from build123d import *

# Parameters (mm, degrees)
F0_W     = 30
F0_H     = 22
F1_DEPTH = 1
F2_R     = 3
F3_R     = 4.5


with BuildPart() as f1:
    # F0 (on Top) → F1 (new body)
    with BuildSketch(Plane.XY):
        Rectangle(F0_W, F0_H)
        Polygon((7.75, 9.5), (13.5, 9.5), (13.5, 3.937851), (13.5, -9.5), (-13.5, -9.5), (-13.5, 3.937851), (-13.5, 9.5), (-7.75, 9.5), align=None, mode=Mode.SUBTRACT)
        Polygon((-13.5, 3.937851), (-7.75, 9.5), (-13.5, 9.5), align=None)
        Polygon((13.5, 3.937851), (13.5, 9.5), (7.75, 9.5), align=None)
    extrude(amount=F1_DEPTH)

    # F2
    f2_edges = [f1.edges().sort_by_distance(p)[0] for p in [
        (13.5, -9.5, 0.5),
        (-13.5, -9.5, 0.5),
    ]]
    fillet(f2_edges, radius=F2_R)

    # F3
    f3_edges = [f1.edges().sort_by_distance(p)[0] for p in [
        (15, -11, 0.5),
        (15, 11, 0.5),
        (-15, -11, 0.5),
        (-15, 11, 0.5),
    ]]
    fillet(f3_edges, radius=F3_R)


solid = f1.part
Work out the finished part from the listing and answer in its coordinate system (mm). A direction names the side the tool comes from. Round coordinates to 2 decimals unless told otherwise and drop trailing zeros. Write each loop counter-clockwise with the first axis right and the second up, starting at its lowest first coordinate (ties: lowest second). Pieces come first, ordered by that corner, then holes. Notation, with made-up numbers: (85.25, 28) -> (142.25, 28) arc R23 cw to (142.25, 60) -> close; hole circle Ø7 at (-1, -38.75). An arc over 180 degrees is marked (long way). Answer as CSV lines item,"result". Start each with the question number.
(1) This flat-tipped pin is pushed along its axis until it touches: pin 1 (12 mm diameter, centred on x = -10.5, y = -6.5, fed in from +Z). Where does it stop, or does it pass through?
(2) The part is cut by section C-C, the plane y = 5. Give the vertices of the cut face in (x, z), then the cut area to 3 significant figures.
(3) The part is cut by section B-B, the plane z = 0.75. Give the vertices of the cut face in (x, y), then the cut area to 3 significant figures.
(4) The part is cut by section A-A, the plane x = 4. Give the vertices of the cut face in (y, z), then the cut area to 3 significant figures.
(5) The mould has two halves that part along X. Classify faces 1 (the flat face through (15, -0.1, 0.5)), 2 (the flat face through (10.58, 6.76, 0.49)), 3 (the flat face through (-15, -0.1, 0.5)): +X half, -X half, draft (parallel to the pull), parting line (faces both ways), or undercut.
(6) A tool of negligible diameter and unlimited length cuts with its end or side. For faces 4 (the cylindrical face through (-12.6, -8.64, 0.51)), 5 (the cylindrical face through (-13.717, -9.647, 0.507)), from which of +Z, -Z, +X, -X, +Y, -Y can it reach the whole face along a straight path? Write none if from no direction.
(7) Find the intervals of material crossed by probe 1 along X at (y, z) = (-4.25, 0.1); probe 2 along Y at (x, z) = (-5.5, 0.5); probe 3 along Y at (x, z) = (-9.25, 0.55), in increasing order.
Output values:
1,pin 1,"stops at z = 1"
2,outline,"(-15, 0) -> (-12.4, 0) -> (-12.4, 1) -> (-15, 1) -> close; (12.4, 0) -> (15, 0) -> (15, 1) -> (12.4, 1) -> close"
2,area,"5.20 mm²"
3,outline,"(-15, -6.5) arc R4.5 ccw to (-10.5, -11) -> (10.5, -11) arc R4.5 ccw to (15, -6.5) -> (15, 6.5) arc R4.5 ccw to (10.5, 11) -> (-10.5, 11) arc R4.5 ccw to (-15, 6.5) -> close; hole (-13.5, -6.5) arc R3 ccw to (-10.5, -9.5) -> (10.5, -9.5) arc R3 ccw to (13.5, -6.5) -> (13.5, 3.94) -> (7.75, 9.5) -> (-7.75, 9.5) -> (-13.5, 3.94) -> close"
3,area,"165 mm²"
4,outline,"(-11, 0) -> (-9.5, 0) -> (-9.5, 1) -> (-11, 1) -> close; (9.5, 0) -> (11, 0) -> (11, 1) -> (9.5, 1) -> close"
4,area,"3.00 mm²"
5,face 1,"+X half"
5,face 2,"undercut"
5,face 3,"-X half"
6,face 4,"+Z, -Z"
6,face 5,"+Z, -Z, -X, -Y"
7,probe 1,"x = -15 to -13.5, 13.5 to 15"
7,probe 2,"y = -11 to -9.5, 9.5 to 11"
7,probe 3,"y = -11 to -9.5, 8.05 to 11"
